Part model, mm, in its own coordinate system. Face numbers are marked on the shaded views. A direction names the side the tool comes from. Coordinates: 2 decimals unless noted, no trailing zeros. Order: outer loops, then holes, each group sorted by start corner. A loop starts at its lowest first (then second) coordinate and runs counter-clockwise, first axis right, second up.
1) Tool access for the marked faces 1, 2 and 3: list every direction of +Z, -Z, +X, -X, +Y, -Y with a clear straight run to the whole face (end or side of a thin tool).
2) Cut at A-A (z = 56.5). List the corners of the cut face in (x, y), and give its area (3 significant figures).
3) Cut at B-B (y = 4.5). List the corners of the cut face in (x, z).
4) Pin check, flat tips, straight feed: pin 1 Ø5 at (x, z) = (-46, 6) entering from +Y; pin 2 Ø1.5 at (y, z) = (6, -22.5) entering from -X; pin 3 Ø3 at (y, z) = (6, 27.5) entering from -X. Stop position of each tip, or through.
5) Cut at C-C (z = -18.5). List the corners of the cut face in (x, y).
6) Wall check: L1, parallel to X at y = -1, z = 52; L2, parallel to X at y = -1, z = -52. Give the ranges that are in metal, low to high.
7) Mould opens along Z. For the marked faces 4 and 5 say: +Z half, -Z half, draft (parallel to the pull), parting line (faces both ways), or undercut.
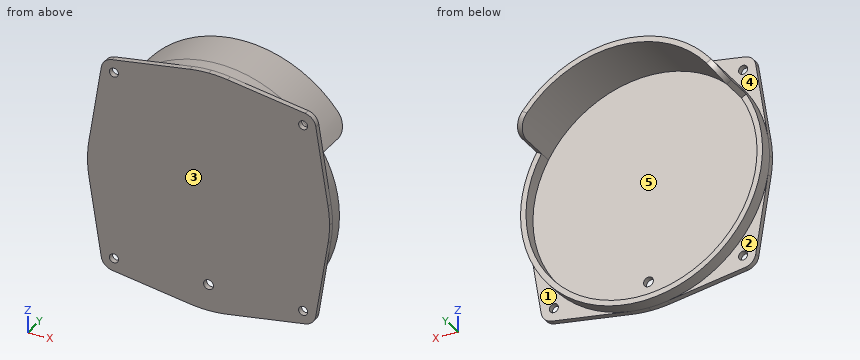
```python
from build123d import *
from build123d.topology import SkipClean

# Parameters (mm, degrees)
SKETCH1_R               = 66.5
SKETCH1_R_2             = 63.5
EXTRUDE_THIN1_DEPTH     = 7
BOSS_EXTRUDE1_DEPTH     = 32
BOSS_EXTRUDE2_DEPTH     = 3
F_10_CLEARANCE_HOLE1_D  = 4.9784
CIRPATTERN1_COUNT       = 4
FILLET1_R               = 10
F_1_4_28_TAPPED_HOLE1_D = 5.4102


with BuildPart() as part:
    # Sketch1 → Extrude-Thin1 (new body)
    with BuildSketch(Plane(origin=(0, 0, 0), x_dir=(1, 0, 0), z_dir=(0, 1, 0))):
        Circle(SKETCH1_R)
        Circle(SKETCH1_R_2, mode=Mode.SUBTRACT)
    extrude(amount=EXTRUDE_THIN1_DEPTH)

    # Sketch2 → Boss-Extrude1 (add)
    with BuildSketch(Plane(origin=(0, 0, 0), x_dir=(1, 0, 0), z_dir=(0, 1, 0))):
        with BuildLine():
            Line((-54.99261314, -31.75), (-57.590689352, -33.25))
            ThreePointArc((-57.590689352, -33.25), (0, -66.5), (57.590689352, -33.25))
            Line((57.590689352, -33.25), (54.99261314, -31.75))
            ThreePointArc((54.99261314, -31.75), (0, -63.5), (-54.99261314, -31.75))
        make_face()
    extrude(amount=BOSS_EXTRUDE1_DEPTH)

    # Sketch3 → Boss-Extrude2 (add)
    with BuildSketch(Plane(origin=(0, 0, 0), x_dir=(1, 0, 0), z_dir=(0, 1, 0))):
        with BuildLine():
            Line((0, 0), (0, 66.5))
            ThreePointArc((0, 66.5), (5.191860277, 66.297017933), (10.352025681, 65.689310883))
            Line((10.352025681, 65.689310883), (53.09577441, 58.953292822))
            ThreePointArc((53.09577441, 58.953292822), (56.977399051, 56.977399051), (58.953292822, 53.09577441))
            Line((58.953292822, 53.09577441), (65.689310883, 10.352025681))
            ThreePointArc((65.689310883, 10.352025681), (66.297017933, 5.191860277), (66.5, 0))
            Line((66.5, 0), (0, 0))
        make_face()
    boss_extrude2 = extrude(amount=-BOSS_EXTRUDE2_DEPTH)

    # #10 Clearance Hole1 (through all)
    with Locations(Plane(origin=(0, 0, 0), x_dir=(1, 0, 0), z_dir=(0, 1, 0))):
        with Locations((52, 52)):
            f_10_clearance_hole1 = Hole(F_10_CLEARANCE_HOLE1_D / 2)

    # CirPattern1: Boss-Extrude2, #10 Clearance Hole1 ×4 about axis
    with SkipClean():  # keep this step's faces unmerged: merging them makes the solid invalid here
        cirpattern1_axis = Axis((0, 0, 0), (0, 1, 0))
        add([boss_extrude2.rotate(cirpattern1_axis, i * 360 / CIRPATTERN1_COUNT) for i in range(1, CIRPATTERN1_COUNT)])
        add([f_10_clearance_hole1.rotate(cirpattern1_axis, i * 360 / CIRPATTERN1_COUNT) for i in range(1, CIRPATTERN1_COUNT)], mode=Mode.SUBTRACT)

    # Fillet1
    fillet1_edges = [part.edges().sort_by_distance(p)[0] for p in [
        (-56.291651246, 32, 32.5),
        (56.291651246, 32, 32.5),
    ]]
    fillet(fillet1_edges, radius=FILLET1_R)

    # 1/4-28 Tapped Hole1 (through all)
    with Locations(Plane(origin=(0, 0, 0), x_dir=(1, 0, 0), z_dir=(0, 1, 0))):
        with Locations((0, 52)):
            Hole(F_1_4_28_TAPPED_HOLE1_D / 2)


solid = part.part
```
Geometry check:
1. face 1: -Z, +X, +Y
1. face 2: -Z, -X, +Y
1. face 3: +Z, -Z, +X, -X, -Y
2. outline: (-57.41, -3) - (57.41, -3) - (57.41, 0) - (35.07, 0) - (35.07, 32) - (28.98, 32) - (28.98, 0) - (-28.98, 0) - (-28.98, 32) - (-35.07, 32) - (-35.07, 0) - (-57.41, 0) - close
2. area: 734 mm2
3. outline: circle Ø133 at (0, 0); hole circle Ø127 at (0, 0)
4. pin 1: stops at y = 0
4. pin 2: stops at x = -62.84
4. pin 3: stops at x = -61.21
5. outline: (-64.41, -3) - (64.41, -3) - (64.41, 0) - (63.87, 0) - (63.87, 7) - (60.75, 7) - (60.75, 0) - (-60.75, 0) - (-60.75, 7) - (-63.87, 7) - (-63.87, 0) - (-64.41, 0) - close
6. L1: x = -59.13 to -54.49, -49.51 to 49.51, 54.49 to 59.13
6. L2: x = -59.13 to -54.49, -49.51 to -2.71, 2.71 to 49.51, 54.49 to 59.13
7. face 4: draft
7. face 5: undercut
